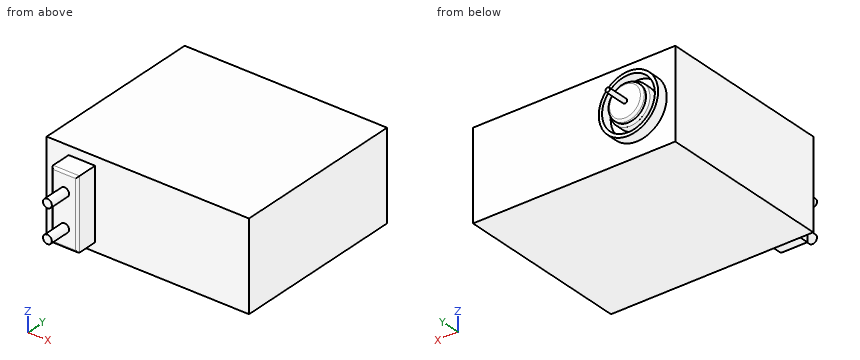
from build123d import *

# Parameters (mm, degrees)
SKETCH1_W           = 46
SKETCH1_H           = 20
BOSS_EXTRUDE1_DEPTH = 40
BOSS_EXTRUDE2_DEPTH = 2.5
SKETCH3_R           = 4
BOSS_EXTRUDE3_DEPTH = 1
FILLET3_R           = 0.5
FILLET4_R           = 0.5
SKETCH5_R           = 0.5
BOSS_EXTRUDE4_DEPTH = 5
SKETCH6_W           = 6
SKETCH6_H           = 16
BOSS_EXTRUDE5_DEPTH = 5
FILLET5_R           = 0.5
SKETCH7_R           = 1
BOSS_EXTRUDE6_DEPTH = 5


with BuildPart() as part:
    # Sketch1 → Boss-Extrude1 (new body)
    with BuildSketch(Plane(origin=(0, 0, 0), x_dir=(1, 0, 0), z_dir=(0, 1, 0))):
        with Locations((-31.181375009, 16.970817206)):
            Rectangle(SKETCH1_W, SKETCH1_H)
    extrude(amount=BOSS_EXTRUDE1_DEPTH)

    # Sketch2 → Boss-Extrude2 (add)
    with BuildSketch(Plane(origin=(0, 40, 0), x_dir=(1, 0, 0), z_dir=(0, 1, 0))):
        with BuildLine():
            ThreePointArc((-49.989558352, 16.970817206), (-45.489558352, 12.470817206), (-40.989558352, 16.970817206))
            Line((-40.989558352, 16.970817206), (-49.989558352, 16.970817206))
        make_face()
        with BuildLine():
            Line((-49.989558352, 16.970817206), (-40.989558352, 16.970817206))
            ThreePointArc((-40.989558352, 16.970817206), (-45.489558352, 21.470817206), (-49.989558352, 16.970817206))
        make_face()
        with BuildLine():
            ThreePointArc((-51.489558352, 16.970817206), (-45.489558352, 22.970817206), (-39.489558352, 16.970817206))
            Line((-39.489558352, 16.970817206), (-38.739558352, 16.970817206))
            ThreePointArc((-38.739558352, 16.970817206), (-45.489558352, 23.720817206), (-52.239558352, 16.970817206))
            Line((-52.239558352, 16.970817206), (-51.489558352, 16.970817206))
        make_face()
        with BuildLine():
            Line((-38.739558352, 16.970817206), (-39.489558352, 16.970817206))
            ThreePointArc((-39.489558352, 16.970817206), (-45.489558352, 10.970817206), (-51.489558352, 16.970817206))
            Line((-51.489558352, 16.970817206), (-52.239558352, 16.970817206))
            ThreePointArc((-52.239558352, 16.970817206), (-45.489558352, 10.220817206), (-38.739558352, 16.970817206))
        make_face()
    extrude(amount=BOSS_EXTRUDE2_DEPTH)

    # Sketch3 → Boss-Extrude3 (add)
    with BuildSketch(Plane(origin=(0, 42.5, 0), x_dir=(1, 0, 0), z_dir=(0, 1, 0))):
        with Locations(Location((-45.489558352, 16.970817206, 0), (0, 0, 270))):
            Circle(SKETCH3_R)
    extrude(amount=BOSS_EXTRUDE3_DEPTH)

    # Fillet3
    fillet3_edges = [part.edges().sort_by_distance(p)[0] for p in [
        (-45.489558352, 43.5, -20.970817206),
    ]]
    fillet(fillet3_edges, radius=FILLET3_R)

    # Fillet4
    fillet4_edges = [part.edges().sort_by_distance(p)[0] for p in [
        (-40.989558352, 42.5, -16.970817206),
    ]]
    fillet(fillet4_edges, radius=FILLET4_R - 0.0001)  # a hair under: the kernel refuses the full size

    # Sketch5 → Boss-Extrude4 (add)
    with BuildSketch(Plane(origin=(0, 43.5, 0), x_dir=(1, 0, 0), z_dir=(0, 1, 0))):
        with Locations(Location((-45.489558352, 16.970817206, 0), (0, 0, 270))):
            Circle(SKETCH5_R)
    extrude(amount=BOSS_EXTRUDE4_DEPTH)

    # Sketch6 → Boss-Extrude5 (add)
    with BuildSketch(Plane.XZ):
        with Locations((-46.181375009, -16.970817206)):
            Rectangle(SKETCH6_W, SKETCH6_H)
    extrude(amount=BOSS_EXTRUDE5_DEPTH)

    # Fillet5
    fillet5_edges = [part.edges().sort_by_distance(p)[0] for p in [
        (-49.181375009, -5, -16.970817206),
        (-46.181375009, -5, -24.970817206),
        (-43.181375009, -5, -16.970817206),
        (-46.181375009, -5, -8.970817206),
    ]]
    fillet(fillet5_edges, radius=FILLET5_R)

    # Sketch7 → Boss-Extrude6 (add)
    with BuildSketch(Plane(origin=(0, -5, 0), x_dir=(-1, 0, 0), z_dir=(0, -1, 0))):
        with Locations(Location((46.181375009, 13.220817206, 0), (0, 0, 90))):
            Circle(SKETCH7_R)
        with Locations(Location((46.181375009, 20.720817206, 0), (0, 0, 90))):
            Circle(SKETCH7_R)
    extrude(amount=BOSS_EXTRUDE6_DEPTH)


solid = part.part
Design review of the part built by this model. Coordinates are the model's own, in mm. Give positions to 0.01 mm unless a question says otherwise; leave off trailing zeros. Write each loop counter-clockwise with the first axis right and the second up, starting at its lowest first coordinate (ties: lowest second). Pieces come first, ordered by that corner, then holes. Notation, with made-up numbers: M 72.5,-40 L 126.5,-40 A27 ccw 126.5,-5 Z; hole C -9,-32.5 d4. An arc over 180 degrees is marked long. Answer as a JSON object with one key per item and string values. Group by question number.
1) We need section B-B (z = -8.25). Give the boundary of the cut face in (x, y).
2) Clearance check with flat-ended pins moving along their axes: pin 1 Ø6 at (x, z) = (-38, -17) entering from -Y; pin 2 Ø1 at (x, y) = (-14, -1.5) entering from +Z; pin 3 Ø1.3 at (x, y) = (-47.5, -1.5) entering from -Z; pin 4 Ø1.3 at (y, z) = (-1.5, -21) entering from -X. State where each tip first meets the part, or that it passes through.
3) We need section A-A (x = -34). Give the boundary of the cut face in (y, z).
4) For line 1 along Y through (x, z) = (-34, -19.75); line 2 along X through (y, z) = (-1.5, -21); line 3 along X through (y, z) = (41, -17.75), list the stretches that pass through material, from the lowest coordinate up.
Answer key:
{
 "1": {"outline": "M -54.18,0 L -8.18,0 L -8.18,40 L -54.18,40 Z"},
 "2": {"pin 1": "stops at y = 0", "pin 2": "passes through", "pin 3": "stops at z = -24.97", "pin 4": "stops at x = -49.18"},
 "3": {"outline": "M 0,-26.97 L 40,-26.97 L 40,-6.97 L 0,-6.97 Z"},
 "4": {"line 1": "y = 0 to 40", "line 2": "x = -49.18 to -43.18", "line 3": "x = -52.19 to -51.44, -49.92 to -41.06, -39.54 to -38.78"}
}
